```python
from build123d import *

# Parameters (mm, degrees)
SKETCH1_W           = 160
SKETCH1_H           = 80
BOSS_EXTRUDE1_DEPTH = 8
SKETCH2_W           = 160
SKETCH2_H           = 80
CUT_EXTRUDE1_DEPTH  = 90.799777283
CUT_EXTRUDE5_DEPTH  = 3.5
SKETCH6_W           = 10.5
SKETCH6_H           = 11
CUT_EXTRUDE6_DEPTH  = 3.5
BOSS_EXTRUDE2_DEPTH = 5
SKETCH13_W          = 202.95713844
SKETCH13_H          = 134.766583704
SKETCH13_W_2        = 22.9414187
SKETCH13_H_2        = 39.597863293
CUT_EXTRUDE7_DEPTH  = 10
CUT_EXTRUDE8_DEPTH  = 3.5
CUT_EXTRUDE9_START  = -2
SKETCH16_W          = 11.5
SKETCH16_H          = 0.936372799
CUT_EXTRUDE9_DEPTH  = 12


with BuildPart() as part:
    # Sketch1 → Boss-Extrude1 (new body)
    with BuildSketch(Plane(origin=(0, 0, 0), x_dir=(1, 0, 0), z_dir=(0, 1, 0))):
        Rectangle(SKETCH1_W, SKETCH1_H)
    extrude(amount=BOSS_EXTRUDE1_DEPTH)

    # Sketch2 → Cut-Extrude1 (cut, through all)
    with BuildSketch(Plane(origin=(0, 8, 0), x_dir=(1, 0, 0), z_dir=(0, 1, 0))):
        Rectangle(SKETCH2_W, SKETCH2_H)
        with BuildLine():
            ThreePointArc((-73.066951559, -31.066887131), (-71.100040398, -34.512464463), (-67.472075966, -36.118271655))
            ThreePointArc((-67.472075966, -36.118271655), (0, -39.461072151), (67.472075966, -36.118271655))
            ThreePointArc((67.472075966, -36.118271655), (71.100040398, -34.512464463), (73.066951559, -31.066887131))
            ThreePointArc((73.066951559, -31.066887131), (76.2, 0), (73.066951559, 31.066887131))
            ThreePointArc((73.066951559, 31.066887131), (71.100040398, 34.512464463), (67.472075966, 36.118271655))
            ThreePointArc((67.472075966, 36.118271655), (0, 39.461072151), (-67.472075966, 36.118271655))
            ThreePointArc((-67.472075966, 36.118271655), (-71.100040398, 34.512464463), (-73.066951559, 31.066887131))
            ThreePointArc((-73.066951559, 31.066887131), (-76.2, 0), (-73.066951559, -31.066887131))
        make_face(mode=Mode.SUBTRACT)
    extrude(amount=-CUT_EXTRUDE1_DEPTH, mode=Mode.SUBTRACT)

    # Sketch3 → Cut-Extrude5 (cut)
    with BuildSketch(Plane(origin=(0, 8, 0), x_dir=(1, 0, 0), z_dir=(0, 1, 0))):
        with BuildLine():
            ThreePointArc((-67.472075966, -36.118271655), (0, -39.461072151), (67.472075966, -36.118271655))
            ThreePointArc((67.472075966, -36.118271655), (71.100040398, -34.512464463), (73.066951559, -31.066887131))
            ThreePointArc((73.066951559, -31.066887131), (76.2, 0), (73.066951559, 31.066887131))
            ThreePointArc((73.066951559, 31.066887131), (71.100040398, 34.512464463), (67.472075966, 36.118271655))
            ThreePointArc((67.472075966, 36.118271655), (0, 39.461072151), (-67.472075966, 36.118271655))
            ThreePointArc((-67.472075966, 36.118271655), (-71.100040398, 34.512464463), (-73.066951559, 31.066887131))
            ThreePointArc((-73.066951559, 31.066887131), (-76.2, 0), (-73.066951559, -31.066887131))
            ThreePointArc((-73.066951559, -31.066887131), (-71.100040398, -34.512464463), (-67.472075966, -36.118271655))
        make_face()
        with BuildLine():
            ThreePointArc((-71.891114808, -30.827287598), (-70.295876764, -33.621778857), (-67.35346279, -34.924148163))
            ThreePointArc((-67.35346279, -34.924148163), (0, -38.261072151), (67.35346279, -34.924148163))
            ThreePointArc((67.35346279, -34.924148163), (70.295876764, -33.621778857), (71.891114808, -30.827287598))
            ThreePointArc((71.891114808, -30.827287598), (75, 0), (71.891114808, 30.827287598))
            ThreePointArc((71.891114808, 30.827287598), (70.295876764, 33.621778857), (67.35346279, 34.924148163))
            ThreePointArc((67.35346279, 34.924148163), (0, 38.261072151), (-67.35346279, 34.924148163))
            ThreePointArc((-67.35346279, 34.924148163), (-70.295876764, 33.621778857), (-71.891114808, 30.827287598))
            ThreePointArc((-71.891114808, 30.827287598), (-75, 0), (-71.891114808, -30.827287598))
        make_face(mode=Mode.SUBTRACT)
    extrude(amount=-CUT_EXTRUDE5_DEPTH, mode=Mode.SUBTRACT)

    # Sketch6 → Cut-Extrude6 (cut)
    with BuildSketch(Plane(origin=(0, 8, 0), x_dir=(1, 0, 0), z_dir=(0, 1, 0))):
        with Locations((0, -38.261072151)):
            Rectangle(SKETCH6_W, SKETCH6_H)
    extrude(amount=-CUT_EXTRUDE6_DEPTH, mode=Mode.SUBTRACT)

    # Sketch5 → Boss-Extrude2 (add, symmetric)
    with BuildSketch(Plane(origin=(0, 0, 0), x_dir=(0, 0, -1), z_dir=(1, 0, 0))):
        Polygon((-33.423273075, 4.5), (-34.597814339, 17.722195507), (-37.101805657, 17.722195507), (-37.101805657, 12.32309307), (-37.944117027, 11.404206925), (-37.101805657, 11.404206925), (-37.101805657, 9.653632864), (-40.188830506, 9.653632864), (-39.785685871, 5.115301729), (-36.101805657, 5.115301729), (-36.101805657, 8.653632864), (-36.101805657, 16.722195507), (-35.51292103, 16.722195507), (-34.427210798, 4.5), align=None)
    extrude(amount=BOSS_EXTRUDE2_DEPTH, both=True)

    # Sketch13 → Cut-Extrude7 (cut)
    with BuildSketch(Plane(origin=(0, 0, 0), x_dir=(1, 0, 0), z_dir=(0, 1, 0))):
        with Locations((1.229729327, -18.57056388)):
            Rectangle(SKETCH13_W, SKETCH13_H)
        with Locations((0, -40.188830507)):
            Rectangle(SKETCH13_W_2, SKETCH13_H_2, mode=Mode.SUBTRACT)
    extrude(amount=CUT_EXTRUDE7_DEPTH, mode=Mode.SUBTRACT)

    # Mirror2: part across plane


with BuildPart() as part_1:
    add(part.part)
    add(part.part.mirror(Plane(origin=(-11.47070935, 10, 20.38989886), x_dir=(1, 0, 0), z_dir=(0, 0, 1))))

    # Sketch14 → Cut-Extrude8 (cut)
    with BuildSketch(Plane(origin=(0, 8, 0), x_dir=(1, 0, 0), z_dir=(0, 1, 0))):
        Polygon((-5.75, -38.24084723), (-5.75, -32.261072151), (5.75, -32.261072151), (5.75, -38.24084723), (5.25, -38.24084723), (5.25, -32.761072151), (-5.25, -32.761072151), (-5.25, -38.24084723), align=None)
        Polygon((5.75, -2.538950489), (5.75, -8.518725569), (-5.75, -8.518725569), (-5.75, -2.538950489), (-5.25, -2.538950489), (-5.25, -8.018725569), (5.25, -8.018725569), (5.25, -2.538950489), align=None)
    extrude(amount=-CUT_EXTRUDE8_DEPTH, mode=Mode.SUBTRACT)

    # Sketch16 → Cut-Extrude9 (cut)
    with BuildSketch(Plane.XY.offset(37.101805657).offset(CUT_EXTRUDE9_START)):
        with Locations((0, 4.0318136)):
            Rectangle(SKETCH16_W, SKETCH16_H)
    cut_extrude9 = extrude(amount=CUT_EXTRUDE9_DEPTH, mode=Mode.SUBTRACT)

    # Mirror3: Cut-Extrude9 across plane
    add(cut_extrude9.mirror(Plane.XY.offset(20.38989886)), mode=Mode.SUBTRACT)


solid = part_1.part
```
Design review of the part built by this model. Coordinates are the model's own, in mm. A direction names the side the tool comes from. Round coordinates to 2 decimals unless told otherwise and drop trailing zeros. Order: outer loops, then holes, each group sorted by start corner. A loop starts at its lowest first (then second) coordinate and runs counter-clockwise, first axis right, second up. Notation, with made-up numbers: M 29,-25 L 86,-25 A25 cw 86,-11 Z; hole C 23,-21 d7. An arc over 180 degrees is marked long. Put each result on its own line as item: value.
Q1. Machinability: for faces 1 (the face through (5, 10, 4)), 2 (the face through (0, 6, 32.261)), 3 (the face through (-5.75, 6, 36)), 4 (the face through (0, 11, 4.678)), which of the approach directions +Z, -Z, +X, -X, +Y, -Y give a long, thin tool a straight path to every point of the face, cutting with its end or side? Answer none if there is none.
Reported:
face 1: -Z, +Y
face 2: +Y
face 3: +Z, +Y
face 4: none
Q2. Insertion check: pin 1 Ø1 at (x, z) = (4.5, 11.5) entering from -Y; pin 2 Ø12 at (x, z) = (-0.5, 17.5) entering from +Y; pin 3 Ø1.4 at (x, y) = (1, 10.5) entering from +Z; pin 4 Ø3.5 at (y, z) = (10.5, 36.5) entering from -X. Each pin has a flat end and moves straight along its axis. Give the tip position at first contact, or say it passes through.
Reported:
pin 1: y = 0
pin 2: y = 8
pin 3: z = 37.1
pin 4: x = -5
Q3. Consider section D-D (z = 20). State the section outline as (x, y) points.
Reported:
outline: M -11.47,0 L 11.47,0 L 11.47,8 L -11.47,8 Z
Q4. Consider section A-A (y = 16). State the section outline as (x, z) points.
Reported:
outline: M -5,3.68 L 5,3.68 L 5,4.68 L -5,4.68 Z; M -5,5.33 L 5,5.33 L 5,6.33 L -5,6.33 Z; M -5,34.44 L 5,34.44 L 5,35.45 L -5,35.45 Z; M -5,36.1 L 5,36.1 L 5,37.1 L -5,37.1 Z
Q5. Consider section B-B (y = 5.75). State the section outline as (x, z) points.
Reported:
outline: M -11.47,2.62 A681.41 ccw -5.75,2.54 L -5.75,8.52 L 5.75,8.52 L 5.75,2.54 A681.41 ccw 11.47,2.62 L 11.47,38.16 A681.41 ccw 5.75,38.24 L 5.75,32.26 L -5.75,32.26 L -5.75,38.24 A681.41 ccw -11.47,38.16 Z; M -5,0.94 L 5,0.94 L 5,4.68 L -5,4.68 Z; M -5,6.24 L 5,6.24 L 5,7.25 L -5,7.25 Z; M -5,33.53 L 5,33.53 L 5,34.54 L -5,34.54 Z; M -5,36.1 L 5,36.1 L 5,39.84 L -5,39.84 Z
Q6. Consider section C-C (x = -8). State the section outline as (y, z) points, and give its area (3 significant figures).
Reported:
outline: M 0,1.37 L 4.5,1.37 L 4.5,2.57 L 8,2.57 L 8,38.21 L 4.5,38.21 L 4.5,39.41 L 0,39.41 Z
area: 296 mm²
Q7. To check wall thickness, follow line 1 (Z direction, x = -3, y = 15); line 2 (Z direction, x = 4.25, y = 5); line 3 (Y direction, x = -4.5, z = 36). State the ranges of each line that lie inside material, in increasing order.
Reported:
line 1: 3.68 to 4.68, 5.42 to 6.42, 34.36 to 35.36, 36.1 to 37.1
line 2: 6.31 to 7.31, 8.52 to 32.26, 33.47 to 34.47
line 3: 0 to 3.56, 16.72 to 17.72
Q8. Draft analysis for pull direction X (two halves, no side actions). For faces 5 (the face through (-5, 10, 4)), 6 (the face through (11.471, 4, 20)), 7 (the face through (0, 9.654, 39)), state which applies: released by +X, released by -X, zero draft, split by the parting line, or undercut.
Reported:
face 5: undercut
face 6: released by +X
face 7: zero draft
